Work out the finished part from the listing and answer in its coordinate system (mm). Face numbers are marked on the shaded views. A direction names the side the tool comes from. Coordinates: 2 decimals unless noted, no trailing zeros. Order: outer loops, then holes, each group sorted by start corner. A loop starts at its lowest first (then second) coordinate and runs counter-clockwise, first axis right, second up. Notation, with made-up numbers: (40, 47) -> (91, 47) arc R27 cw to (91, 70) -> close; hole circle Ø10 at (44.5, -10.75). An arc over 180 degrees is marked (long way). Write item = value, one per line. Start each with the question number.
Q1. Straight lines are drawn through the part: L1, parallel to Y at x = 9, z = 22.5; L2, parallel to Y at x = 7.5, z = 16.25; L3, parallel to X at y = -46.5, z = 12.5. For each, find the intervals that lie inside material, in ascending order. Write a range as from..to.
Q2. The part is cut by section A-A, the plane z = 16.5. Count the separate pieces of the cut face and the enclosed holes in it, plus the area to 3 significant figures.
Q3. For a pull along X with two mould halves and no side action, classify the marked faces 1, 2, 3 and 4 as +X half, -X half, draft (parallel to the pull), parting line (faces both ways), or undercut.
Q4. Flat-ended cylindrical pins translate along their axes: pin 1 (3 mm diameter, centred on x = 45.5, z = 18.5, fed in from +Y); pin 2 (1 mm diameter, centred on y = 55, z = 18.5, fed in from +X); pin 3 (8 mm diameter, centred on x = 27.5, z = 4.5, fed in from +Y); pin 4 (11 mm diameter, centred on x = 19.05, y = 44.45, fed in from -Z). Find the tip coordinate at first contact, or state that the pin passes through.
Q5. The part is cut by section D-D, the plane z = 6.75. Determine the outline of the cut face in (x, y), plus the area to 3 significant figures.
Q6. Which of the six approach directions +Z, -Z, +X, -X, +Y, -Y give full straight-line access (tool end or side, diameter ignored) to the marked faces 5 and 6?
Q7. The part is cut by section C-C, the plane x = 44.45. Determine the outline of the cut face in (y, z).
Q8. The part is cut by section B-B, the plane y = 0. Determine the outline of the cut face in (x, z).
```python
from build123d import *

# Parameters (mm, degrees)
F1_DEPTH = 25.4
F2_R     = 4.7675
F3_DEPTH = 12.7


with BuildPart() as f1:
    # F0 (on Top) → F1 (new body)
    with BuildSketch(Plane.XY):
        with BuildLine():
            Line((0, -19.05), (0, -69.85))
            ThreePointArc((0, -69.85), (69.85, 0), (0, 69.85))
            Line((0, 69.85), (0, 19.05))
            ThreePointArc((0, 19.05), (19.05, 0), (0, -19.05))
        make_face()
    extrude(amount=F1_DEPTH)

    # F2 (on face) → F3 (cut)
    with BuildSketch(Plane.XY.offset(25.4)):
        with Locations((19.05, 44.45)):
            Circle(F2_R)
        with Locations((19.05, -44.45)):
            Circle(F2_R)
        with Locations((44.45, 0)):
            Circle(F2_R)
    extrude(amount=-F3_DEPTH, mode=Mode.SUBTRACT)


solid = f1.part
```
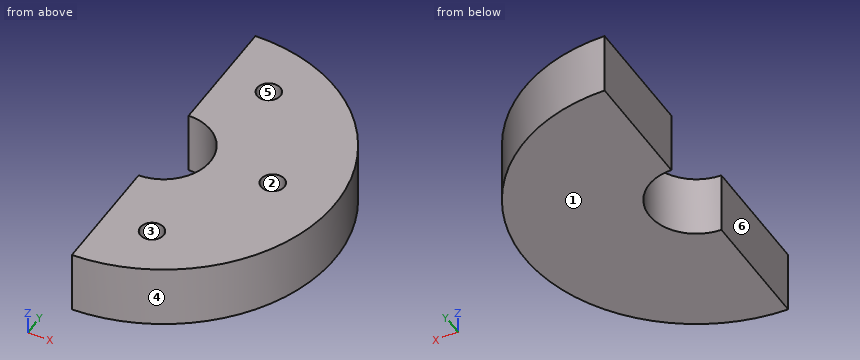
Model answer:
q1.L1 = -69.27..-16.79, 16.79..69.27
q1.L2 = -69.45..-17.51, 17.51..69.45
q1.L3 = 0..52.12
q2.separate_pieces = 1
q2.enclosed_holes = 3
q2.area = 6,880 mm2
q3.face_1 = draft
q3.face_2 = undercut
q3.face_3 = undercut
q3.face_4 = +X half
q4.pin_1 = 54.25
q4.pin_2 = 43.69
q4.pin_3 = 65.78
q4.pin_4 = 0
q5.outline = (0, -69.85) arc R69.85 ccw to (0, 69.85) -> (0, 19.05) arc R19.05 cw to (0, -19.05) -> close
q5.area = 7,090 mm2
q6.face_5 = +Z
q6.face_6 = +Z, -Z, -X, +Y, -Y
q7.outline = (-53.88, 0) -> (53.88, 0) -> (53.88, 25.4) -> (4.77, 25.4) -> (4.77, 12.7) -> (-4.77, 12.7) -> (-4.77, 25.4) -> (-53.88, 25.4) -> close
q8.outline = (19.05, 0) -> (69.85, 0) -> (69.85, 25.4) -> (49.22, 25.4) -> (49.22, 12.7) -> (39.68, 12.7) -> (39.68, 25.4) -> (19.05, 25.4) -> close
